The model under review builds one solid part; all positions refer to its coordinate system, in mm. A direction names the side the tool comes from. Give positions to 0.01 mm unless a question says otherwise; leave off trailing zeros. Order: outer loops, then holes, each group sorted by start corner. A loop starts at its lowest first (then second) coordinate and runs counter-clockwise, first axis right, second up.
```python
from build123d import *

# Parameters (mm, degrees)
SKETCH1_W                                            = 20
SKETCH1_H                                            = 35
BOSS_EXTRUDE1_DEPTH                                  = 20
CBORE_FOR_M3_HEXAGON_SOCKET_HEAD_CAP_SCR_D           = 3.2
CBORE_FOR_M3_HEXAGON_SOCKET_HEAD_CAP_SCR_CBORE_D     = 6
CBORE_FOR_M3_HEXAGON_SOCKET_HEAD_CAP_SCR_CBORE_DEPTH = 3.4
TAP_DRILL_FOR_M3_TAP1_D                              = 2.5
TAP_DRILL_FOR_M3_TAP1_DEPTH                          = 5
TAP_DRILL_FOR_M3_TAP1_TIP                            = 0.751075774


with BuildPart() as part:
    # Sketch1 → Boss-Extrude1 (new body)
    with BuildSketch(Plane.XY):
        Rectangle(SKETCH1_W, SKETCH1_H)
    extrude(amount=BOSS_EXTRUDE1_DEPTH)

    # CBORE for M3 Hexagon socket head cap screws1 (through all)
    with Locations(Plane(origin=(0, 9.5, 20), x_dir=(1, 0, 0), z_dir=(0, 0, 1))):
        with Locations((0, 0), (0, -19)):
            CounterBoreHole(CBORE_FOR_M3_HEXAGON_SOCKET_HEAD_CAP_SCR_D / 2, CBORE_FOR_M3_HEXAGON_SOCKET_HEAD_CAP_SCR_CBORE_D / 2, CBORE_FOR_M3_HEXAGON_SOCKET_HEAD_CAP_SCR_CBORE_DEPTH)

    # Tap Drill for M3 Tap1
    with Locations(Plane(origin=(0, 17.5, 0), x_dir=(1, 0, 0), z_dir=(0, 1, 0))):
        with Locations((0, -10)):
            Hole(TAP_DRILL_FOR_M3_TAP1_D / 2, depth=TAP_DRILL_FOR_M3_TAP1_DEPTH)
            with Locations((0, 0, -(TAP_DRILL_FOR_M3_TAP1_DEPTH + TAP_DRILL_FOR_M3_TAP1_TIP / 2))):  # 118° drill point
                Cone(0, TAP_DRILL_FOR_M3_TAP1_D / 2, TAP_DRILL_FOR_M3_TAP1_TIP, mode=Mode.SUBTRACT)


solid = part.part
```
1. Take a section at B-B (z = 5). Write out the cut boundary in (x, y).
2. Draft analysis for pull direction X (two halves, no side actions). For faces 1 (the cylindrical face through (-3, 9.6, 18.3)), 2 (the flat face through (-10, 0, 10)), 3 (the flat face through (0, -17.5, 10)), state which applies: pulls with the +X half, pulls with the -X half, needs draft (parallel to the pull), parting line crosses it, or undercut.
3. Take a section at C-C (y = -8.5). Write out the cut boundary in (x, z), and give its area (3 significant figures).
4. Take a section at D-D (z = 18). Write out the cut boundary in (x, y), and give its area (3 significant figures).
5. Insertion check: pin 1 (1 mm diameter, centred on x = -2, y = -6, fed in from -Z); pin 2 (1.8 mm diameter, centred on x = 0, y = -8, fed in from +Z); pin 3 (3 mm diameter, centred on x = 0, y = 9.5, fed in from -Z). Each pin has a flat end and moves straight along its axis. Give the tip position at first contact, or say it passes through.
6. To check wall thickness, follow line 1 (Y direction, x = 0, z = 18.25); line 2 (X direction, y = 14.9, z = 10); line 3 (Y direction, x = 0, z = 11.5). State the ranges of each line that lie inside material, in increasing order.
7. Take a section at A-A (y = 9.5). Write out the cut boundary in (x, z), and give its area (3 significant figures).
8. For faces 4 (the flat face through (0, 0, 0)), 5 (the flat face through (1, 8, 16.6)), 6 (the cylindrical face through (-0.672, 14.965, 8.946)), list the 3-axis set-ups (+Z, -Z, +X, -X, +Y, -Y) from which the entire face can be reached by the end or side of a thin tool; tool diameter is ignored.
Answer:
1. outline: (-10, -17.5) - (10, -17.5) - (10, 17.5) - (-10, 17.5) - close; hole circle Ø3.2 at (0, -9.5); hole circle Ø3.2 at (0, 9.5)
2. face 1: undercut
2. face 2: pulls with the -X half
2. face 3: needs draft
3. outline: (-10, 0) - (-1.25, 0) - (-1.25, 16.6) - (-2.83, 16.6) - (-2.83, 20) - (-10, 20) - close; (1.25, 0) - (10, 0) - (10, 20) - (2.83, 20) - (2.83, 16.6) - (1.25, 16.6) - close
3. area: 339 mm2
4. outline: (-10, -17.5) - (10, -17.5) - (10, 17.5) - (-10, 17.5) - close; hole circle Ø6 at (0, -9.5); hole circle Ø6 at (0, 9.5)
4. area: 643 mm2
5. pin 1: stops at z = 0
5. pin 2: stops at z = 16.6
5. pin 3: passes through
6. line 1: y = -17.5 to -12.5, -6.5 to 6.5, 12.5 to 17.5
6. line 2: x = -10 to -1.25, 1.25 to 10
6. line 3: y = -17.5 to -11.1, -7.9 to 7.9, 11.1 to 17.5
7. outline: (-10, 0) - (-1.6, 0) - (-1.6, 16.6) - (-3, 16.6) - (-3, 20) - (-10, 20) - close; (1.6, 0) - (10, 0) - (10, 20) - (3, 20) - (3, 16.6) - (1.6, 16.6) - close
7. area: 326 mm2
8. face 4: -Z, +X, -X, +Y, -Y
8. face 5: +Z
8. face 6: +Y
